Autodesk Inventor part; units mm, degrees
ref_plane "YZ Plane" through (0, 0, 0) normal (1, 0, 0) x (0, 1, 0)
ref_plane "XZ Plane" through (0, 0, 0) normal (0, 1, 0) x (-1, 0, 0)
ref_plane "XY Plane" through (0, 0, 0) normal (0, 0, 1) x (1, 0, 0)
sketch "Sketch1" plane through (0, 0, 0) normal (0, 1, 0) x (-1, 0, 0)
  circle A0 centre (0, 0) radius 10
  circle A1 centre (11.9909, 79.0327) radius 10 construction
  circle A2 centre (11.9909, 79.0327) radius 10.5
  circle A3 centre (-8.6473, 36.4616) radius 22.3944 construction
  circle A4 centre (-8.6473, 36.4616) radius 25.3944
  circle A5 centre (6.4474, -27.1859) radius 9.5
  arc A6 (1.4403, 93.6164) -> (29.9753, 79.7828) centre (11.9909, 79.0327) ccw construction
  arc A7 (-42.203, 13.9734) -> (31.4334, 31.4371) centre (-8.6473, 36.4616) ccw construction
  arc A8 (23.8115, -29.3627) -> (-8.0899, -36.9284) centre (6.4474, -27.1859) ccw construction
  line L0 (-8.0899, -36.9284) -> (-42.203, 13.9734)
  line L1 (23.8115, -29.3627) -> (31.4334, 31.4371)
  line L2 (-32.3242, 69.1894) -> (1.4403, 93.6164)
  line L3 (31.712, 38.145) -> (29.9753, 79.7828)
  arc A9 (29.9753, 79.7828) -> (1.4403, 93.6164) centre (11.9909, 79.0327) ccw
  arc A10 (-32.3242, 69.1894) -> (-42.203, 13.9734) centre (-8.6473, 36.4616) ccw
  arc A11 (31.712, 38.145) -> (-32.3242, 69.1894) centre (-8.6473, 36.4616) ccw construction
  arc A12 (31.4334, 31.4371) -> (31.712, 38.145) centre (-8.6473, 36.4616) ccw
  arc A13 (-8.0899, -36.9284) -> (23.8115, -29.3627) centre (6.4474, -27.1859) ccw
  dimension "d0" = 20
  dimension "d5" = 0.5
  dimension "d6" = 3
  dimension "d7" = 8
  dimension "d8" = 15
  dimension "d9" = 8
extrude "Extrusion1" add sketch "Sketch1" along normal blind 3
sketch "Sketch2" plane through (0, 0, 0) normal (0, -1, 0) x (1, 0, 0)
  circle A0 centre (35.2337, 17.429) radius 2.2
  circle A1 centre (-20.9595, 57.0259) radius 2.2
  circle A2 centre (13.6085, 72.7436) radius 2.2
  point P0 (0, 0)
  dimension "d12" = 4.4
  dimension "d13" = 4.4
  dimension "d14" = 4.4
extrude "Extrusion2" cut sketch "Sketch2" against normal blind 5
sketch "Sketch3" plane through (0, 0, 0) normal (0, -1, 0) x (1, 0, 0)
  circle A0 centre (35.893, -3.2614) radius 2.75
  circle A1 centre (35.893, -3.2614) radius 6
  circle A2 centre (49.8895, 56.3777) radius 2.75
  circle A3 centre (49.8895, 56.3777) radius 6
  circle A4 centre (-36.0964, 28.5483) radius 2.75
  circle A5 centre (-36.0964, 28.5483) radius 6
  circle A6 centre (-33.3464, 74.8865) radius 2.75
  circle A7 centre (-33.3464, 74.8865) radius 6
  point P0 (0, 0)
  dimension "d18" = 5.5
  dimension "d19" = 12
  dimension "d20" = 5.5
  dimension "d21" = 12
  dimension "d22" = 5.5
  dimension "d23" = 12
  dimension "d24" = 5.5
  dimension "d25" = 12
extrude "Extrusion3" add sketch "Sketch3" against normal blind 3
fillet "Fillet1" radius 2 6 edges at (29.978, 1.5, -4.268) (34.5756, 1.5, 2.5922) (46.0191, 1.5, 51.793) (43.8922, 1.5, 56.1973) (-30.3974, 1.5, 69.6612) (-30.7339, 1.5, 25.857)
sketch "Sketch4" plane through (0, 0, 0) normal (0, -1, 0) x (1, 0, 0)
  circle A0 centre (23.213, -10.311) radius 2.413
  circle A1 centre (-23.213, 10.311) radius 2.413
  circle A2 centre (-20.5361, -14.9476) radius 2.413
  circle A3 centre (23.213, -10.311) radius 2.75
  circle A4 centre (-23.213, 10.311) radius 2.75
  circle A5 centre (-20.5361, -14.9476) radius 2.75
  point P0 (0, 0)
  dimension "d29" = 5.5
  dimension "d30" = 5.5
  dimension "d31" = 5.5
extrude "Extrusion4" cut sketch "Sketch4" against normal through all contours A0 | A1 | A2 | A3 | A4 | A5
sketch "Sketch5" plane through (0, 0, 0) normal (0, -1, 0) x (1, 0, 0)
  circle A0 centre (23.213, -10.311) radius 2.75
  circle A1 centre (23.213, -10.311) radius 2.75
  circle A2 centre (23.213, -10.311) radius 6
  point P0 (0, 0)
  point P1 (25.9625, -10.2598)
  point P2 (24.2108, -12.8736)
  dimension "d34" = 12
extrude "Extrusion5" add sketch "Sketch5" against normal blind 3 contours A0 | A2
fillet "Fillet2" radius 2 2 edges at (28.1941, 1.5, -6.966) (21.9914, 1.5, -16.1853)
sketch "Sketch6" plane through (0, 3, 0) normal (0, 1, 0) x (1, 0, 0)
  circle A0 centre (-11.9909, -79.0327) radius 10.5
  circle A1 centre (3.0091, -79.0327) radius 1.65
  line L0 (3.0091, -79.0327) -> (-11.9909, -79.0327) construction
  circle A2 centre (-19.4909, -66.0423) radius 1.65
  circle A3 centre (-19.4909, -92.023) radius 1.65
  point P0 (0, 0)
  dimension "d38" = 3.3
  dimension "d39" = 15
  dimension "d42" = 360
extrude "Extrusion6" cut sketch "Sketch6" against normal blind 10 contours A1 | A2 | A3
properties part number "Motor Mount Plate" material "Aluminum 6061"
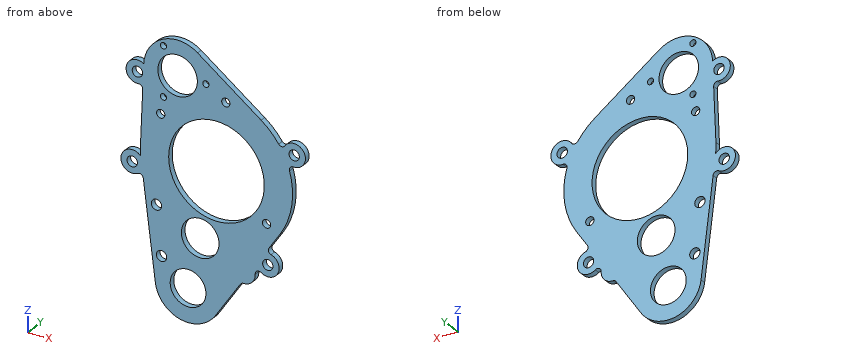
Geometry: final body of the model. Coordinates: model frame, mm. Round coordinates to 2 decimals unless told otherwise and drop trailing zeros. Order: outer loops, then holes, each group sorted by start corner. A loop starts at its lowest first (then second) coordinate and runs counter-clockwise, first axis right, second up.
Q1. Material intervals for probe 1 along X at (y, z) = (1.65, -3); probe 2 along X at (y, z) = (0.95, 26.5); probe 3 along X at (y, z) = (0.4, 36.5), sorted ascending.
Result sheet:
probe 1: x = -27.12 to -9.54, 9.54 to 33.16, 38.63 to 41.89
probe 2: x = -41.74 to -37.93, -34.26 to -14.71, 32.01 to 47.79
probe 3: x = -31.75 to -16.75, 34.04 to 49.04
Q2. Pin query (flat end, axial travel): pin 1 (2 mm diameter, centred on x = -14.5, z = 66, fed in from -Y); pin 2 (1.5 mm diameter, centred on x = 29, y = 2, fed in from -Z); pin 3 (1 mm diameter, centred on x = -27.5, y = 0.5, fed in from +Z). Return the tip coordinate at first contact, or that it passes through.
Result sheet:
pin 1: stops at y = 0
pin 2: stops at z = -13.57
pin 3: stops at z = 88.97
Q3. Section B-B, the plane y = 1.3. Give the number of separate pieces and of enclosed holes in the cut face, and give its area (3 significant figures).
Result sheet:
separate pieces: 1
enclosed holes: 16
area: 5,370 mm2
Q4. Section A-A, the plane x = -4. Output: boundary loops of the cut face in (y, z).
Result sheet:
outline: (0, -44.51) - (3, -44.51) - (3, -36.37) - (0, -36.37) - close; (0, -18.01) - (3, -18.01) - (3, -9.17) - (0, -9.17) - close; (0, 9.17) - (3, 9.17) - (3, 14.44) - (0, 14.44) - close; (0, 58.48) - (3, 58.48) - (3, 72.22) - (0, 72.22) - close; (0, 85.84) - (3, 85.84) - (3, 95.16) - (0, 95.16) - close
